Autodesk Fusion 360 part; units mm, degrees
sketch "Sketch1" plane through (0, 0, 0) normal (0, 0, 1) x (1, 0, 0)
  line L0 (0, 0) -> (90, 0)
  line L1 (90, 0) -> (90, 120)
  line L2 (90, 120) -> (0, 120)
  line L3 (0, 120) -> (0, 0)
  circle A0 centre (5, 35) radius 2
  circle A1 centre (5, 85) radius 2
  dimension "d1" = 90
  dimension "d2" = 120
  dimension "d4" = 4
  dimension "d9" = 35
  dimension "d10" = 5
  dimension "d43" = 0
  dimension "d44" = 50
extrude "Extrude1" add sketch "Sketch1" along normal blind 2
sketch "Sketch2" plane through (0, 0, 2) normal (0, 0, 1) x (-1, 0, 0)
  circle A0 centre (-5, -35) radius 2
  line L0 (0, -120) -> (0, 0)
  line L1 (0, 0) -> (-90, 0)
  line L2 (-90, 0) -> (-90, -120)
  line L3 (-90, -120) -> (0, -120)
  line L4 (-90, 0) -> (-10, 0)
  line L5 (-10, 0) -> (-10, -120)
  line L6 (-10, -120) -> (-90, -120)
  line L7 (-90, -120) -> (-90, 0)
  line L8 (-10, -120) -> (-90, -120)
  line L9 (-90, -120) -> (-90, -118)
  line L10 (-90, -118) -> (-10, -118)
  line L11 (-10, -118) -> (-10, -120)
  line L12 (-10, -120) -> (-12, -120)
  line L13 (-12, -120) -> (-12, 0)
  line L14 (-12, 0) -> (-10, 0)
  line L15 (-10, 0) -> (-10, -120)
  line L16 (-90, 0) -> (-10, 0)
  line L17 (-10, 0) -> (-10, -2)
  line L18 (-10, -2) -> (-90, -2)
  line L19 (-90, -2) -> (-90, 0)
  line L20 (-90, 0) -> (-88, 0)
  line L21 (-88, 0) -> (-88, -120)
  line L22 (-88, -120) -> (-90, -120)
  line L23 (-90, -120) -> (-90, 0)
  circle A1 centre (-5, -85) radius 2
  dimension "d13" = 2
  dimension "d14" = 2
  dimension "d15" = 120
  dimension "d16" = 2
  dimension "d17" = 2
extrude "Extrude2" add sketch "Sketch2" along normal blind 30 contours L3 L5 L6 L8 L10 L11 L12 L13 L15 | L1 L4 L5 L13 L14 L15 L16 L17 L18 | L3 L6 L8 L10 L13 L21 | L5 L10 L13 L15 L18 | L1 L4 L13 L16 L18 L21 | L2 L3 L6 L7 L8 L9 L10 L21 L22 L23 | L1 L2 L4 L7 L16 L18 L19 L20 L21 L23 | L2 L7 L10 L18 L21 L23
sketch "Sketch3" plane through (0, 120, 0) normal (0, 1, 0) x (-1, 0, 0)
  line L0 (-90, 0) -> (0, 0)
  line L1 (0, 0) -> (0, 2)
  line L2 (0, 2) -> (-10, 2)
  line L3 (-10, 2) -> (-10, 32)
  line L4 (-10, 32) -> (-90, 32)
  line L5 (-90, 32) -> (-90, 0)
  circle A0 centre (-70, 42) radius 18
  line L6 (-88, 2) -> (-88, 32)
  dimension "d20" = 36
  dimension "d26" = 18
  dimension "d39" = 42
sketch "Sketch4" plane through (0, 0, 0) normal (0, -1, 0) x (1, 0, 0)
  line L0 (0, 0) -> (90, 0)
  line L1 (90, 0) -> (90, 32)
  line L2 (90, 32) -> (10, 32)
  line L3 (10, 32) -> (10, 2)
  line L4 (10, 2) -> (0, 2)
  line L5 (0, 2) -> (0, 0)
  circle A0 centre (30, 42) radius 18
  line L6 (12, 2) -> (12, 32)
  dimension "d28" = 36
  dimension "d29" = 18
  dimension "d40" = 42
hole "Hole1" at (30, 0, 42) direction (0, 1, 0) diameter 36 depth 4 tip angle 180
hole "Hole2" at (70, 120, 42) direction (0, -1, 0) diameter 36 depth 20 tip angle 118
Input: part model. Units: mm. Frame: model coordinates. A direction names the side the tool comes from. Round coordinates to 2 decimals unless told otherwise and drop trailing zeros. Write each loop counter-clockwise with the first axis right and the second up, starting at its lowest first coordinate (ties: lowest second). Pieces come first, ordered by that corner, then holes.
1) Cut plane A-A (x = 5). Return the cut outline in (y, z), then the cut area to 3 significant figures.
2) Cut plane C-C (z = 13). Return the cut outline in (x, y).
3) Contact query for flat-ended pins moving along their axis: P1, Ø10, axis at x = 36, y = 40.5, coming from the -Z side; P2, Ø5, axis at x = 5, y = 85, coming from the +Z side; P3, Ø2, axis at y = 33.5, z = 19, coming from the -X side. Output: stop coordinate, or through.
4) Cut plane B-B (y = 85). Return the cut outline in (x, z), then the cut area to 3 significant figures.
5) Ray query, L1, parallel to Y at x = 5, z = 0.4; L2, parallel to X at y = 8, z = 2.5; L3, parallel to Y at x = 82.5, z = 7.5. Return the intervals inside material, ascending.
6) Cut plane D-D (y = 105.5). Return the cut outline in (x, z), then the cut area to 3 significant figures.
7) Reachability of faces 1 (the flat face through (46, 120, 16)), 2 (the cylindrical face through (30, 1, 24)), 3 (the cylindrical face through (70, 119, 24)), 4 (the flat face through (12, 61, 17)), 5 (the flat face through (5, 61, 2)) from +Z, -Z, +X, -X, +Y, -Y: full face, straight path, thin tool, end or side. Return the list, or none.
8) Draft query along X for faces 6 (the flat face through (10, 59, 17)), 7 (the flat face through (11, 55, 32)), 8 (the cylindrical face through (5, 83, 1)). Return one class per face: pulls with the +X half, pulls with the -X half, needs draft (parallel to the pull), parting line crosses it, or undercut.
Geometry says:
1. outline: (0, 0) - (33, 0) - (33, 2) - (0, 2) - close; (37, 0) - (83, 0) - (83, 2) - (37, 2) - close; (87, 0) - (120, 0) - (120, 2) - (87, 2) - close
1. area: 224 mm2
2. outline: (10, 0) - (90, 0) - (90, 120) - (10, 120) - close; hole (12, 2) - (88, 2) - (88, 118) - (12, 118) - close
3. P1: stops at z = 0
3. P2: stops at z = 2
3. P3: stops at x = 10
4. outline: (0, 0) - (3, 0) - (3, 2) - (0, 2) - close; (7, 0) - (90, 0) - (90, 32) - (88, 32) - (88, 2) - (12, 2) - (12, 32) - (10, 32) - (10, 2) - (7, 2) - close
4. area: 292 mm2
5. L1: y = 0 to 33, 37 to 83, 87 to 120
5. L2: x = 10 to 12, 88 to 90
5. L3: y = 0 to 2, 118 to 120
6. outline: (0, 0) - (90, 0) - (90, 32) - (88, 32) - (88, 2) - (12, 2) - (12, 32) - (10, 32) - (10, 2) - (0, 2) - close
6. area: 300 mm2
7. face 1: +Z, -Z, +X, -X, +Y
7. face 2: +Z, -Y
7. face 3: +Z, +Y
7. face 4: +Z
7. face 5: +Z, -X, +Y, -Y
8. face 6: pulls with the -X half
8. face 7: needs draft
8. face 8: undercut
